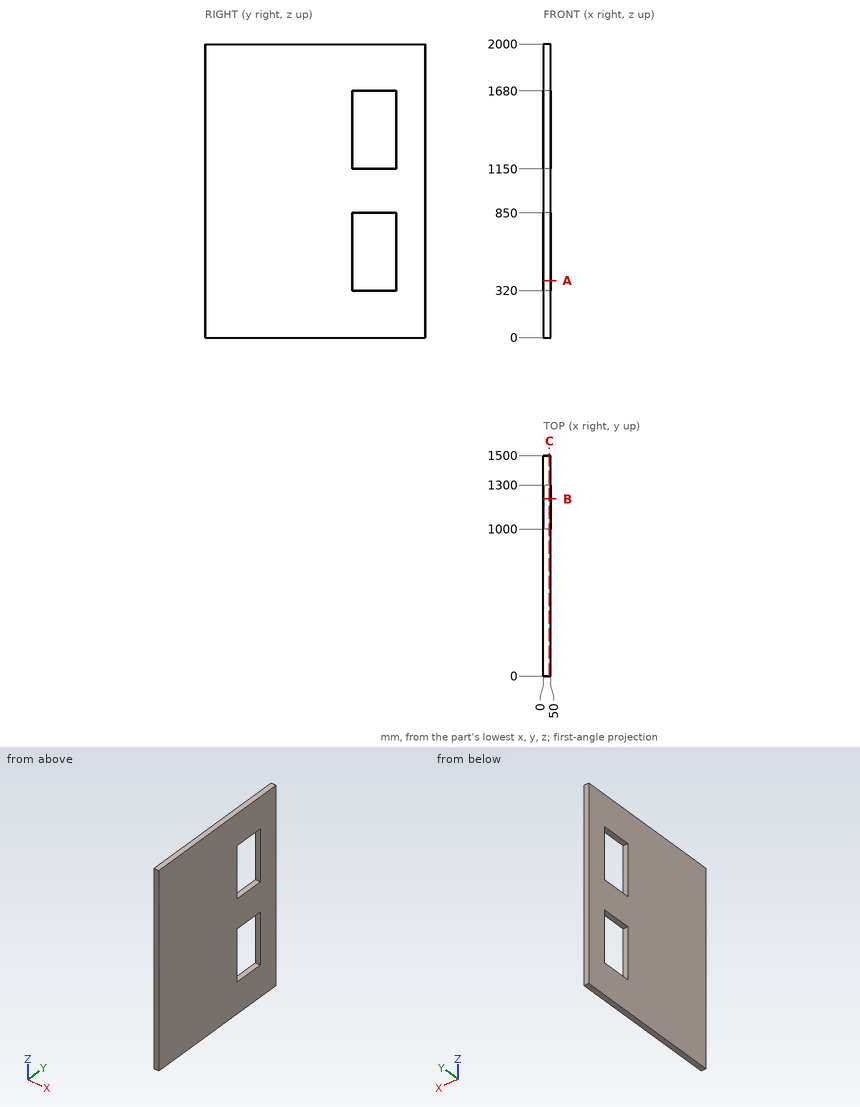
Geometry: see drawing. Coordinates: mm, zero at the bounding-box minimum. Coordinates: 2 decimals unless noted, no trailing zeros. Loops run counter-clockwise (first coordinate to the right, second up) from the corner with the lowest first, then second, coordinate; pieces in that order, holes last. Notation, with made-up numbers: (41, -9) - (49, -9) arc R37 ccw to (49, 28) - close; hole circle Ø4 at (24, 32.25). An arc over 180 degrees is marked (long way). Answer in a Markdown table with one row per item.
(1) Cut plane A-A on z = 388.5. Output: boundary loops of the cut face in (x, y).
Model answer:
| item | result |
|---|---|
| outline | (0, 0) - (50, 0) - (50, 1000) - (0, 1000) - close; (0, 1300) - (50, 1300) - (50, 1500) - (0, 1500) - close |
(2) Cut plane C-C on x = 40.5. Output: boundary loops of the cut face in (y, z).
Model answer:
| item | result |
|---|---|
| outline | (0, 0) - (1500, 0) - (1500, 2000) - (0, 2000) - close; hole (1000, 320) - (1300, 320) - (1300, 850) - (1000, 850) - close; hole (1000, 1150) - (1300, 1150) - (1300, 1680) - (1000, 1680) - close |
(3) Cut plane B-B on y = 1206. Output: boundary loops of the cut face in (x, z).
Model answer:
| item | result |
|---|---|
| outline | (0, 0) - (50, 0) - (50, 320) - (0, 320) - close; (0, 850) - (50, 850) - (50, 1150) - (0, 1150) - close; (0, 1680) - (50, 1680) - (50, 2000) - (0, 2000) - close |
(4) Material intervals for L1, parallel to Z at x = 35.5, y = 1080; L2, parallel to Y at x = 45, z = 1459.5, sorted ascending. Write a range as from..to.
Model answer:
| item | result |
|---|---|
| L1 | z = 0..320, 850..1150, 1680..2000 |
| L2 | y = 0..1000, 1300..1500 |
